Autodesk Fusion 360 part; units mm, degrees
sketch "Sketch1" plane through (0, 0, 0) normal (0, 1, 0) x (1, 0, 0)
  circle A0 centre (0, 0) radius 17 construction
  line L0 (-50, -17) -> (32, -17) construction
  line L1 (32, -17) -> (32, 83) construction
  line L2 (32, 83) -> (-50, 83) construction
  line L3 (-50, 83) -> (-50, -17) construction
  line L4 (-52.028, -78) -> (57.972, -78)
  line L5 (57.972, -78) -> (57.972, -8)
  line L6 (57.972, -8) -> (-52.028, -8)
  line L7 (57.972, -8) -> (32.972, -8)
  line L8 (32.972, -8) -> (32.972, -33)
  line L9 (32.972, -33) -> (57.972, -33)
  line L10 (57.972, -33) -> (57.972, -8)
  line L11 (-52.028, -78) -> (-52.028, -8)
  line L12 (-52.028, -8) -> (57.972, -8)
  line L13 (57.972, -8) -> (57.972, -33)
  line L14 (32.972, -8) -> (57.972, -8)
  line L15 (57.972, -8) -> (57.972, 42)
  line L16 (57.972, 42) -> (32.972, 42)
  line L17 (32.972, 42) -> (32.972, -8)
  line L18 (57.972, 42) -> (-52.028, 42)
  line L19 (-52.028, 42) -> (-52.028, 17)
  line L20 (-52.028, 17) -> (57.972, 17)
  line L21 (57.972, 17) -> (57.972, 42)
  line L22 (-52.028, 17) -> (-52.028, 2)
  line L23 (-52.028, 2) -> (-27.028, 2)
  line L24 (-27.028, 2) -> (-27.028, 17)
  circle A1 centre (-37.028, -63) radius 2.5
  circle A2 centre (42.972, -63) radius 2.5
  circle A3 centre (2.972, -28) radius 2.5
  line L25 (2.972, -78) -> (2.972, -8) construction
  dimension "d1" = 34
  dimension "d2" = 82
  dimension "d3" = 32
  dimension "d4" = 100
  dimension "d5" = 25
  dimension "d6" = 25
  dimension "d7" = 110
  dimension "d8" = 70
  dimension "d9" = 25
  dimension "d10" = 50
  dimension "d11" = 110
  dimension "d12" = 25
  dimension "d13" = 15
  dimension "d14" = 25
  dimension "d15" = 5
  dimension "d16" = 5
  dimension "d17" = 5
  dimension "d18" = 50
  dimension "d19" = 15
  dimension "d20" = 15
  dimension "d21" = 15
  dimension "d22" = 15
extrude "Extrude1" add sketch "Sketch1" along normal blind 10 contours L4 L5 L6 L8 L9 L11 L12 | L5 L6 L7 L8 L9 L10 L12 L13 L14
extrude "Extrude2" add sketch "Sketch1" against normal blind 25 contours L5 L6 L7 L8 L9 L10 L12 L13 L14
extrude "Extrude3" add sketch "Sketch1" along normal blind 25 from surface at -50 contours L5 L6 L7 L8 L9 L10 L12 L13 L14 | L6 L7 L12 L14 L15 L17 L20 | L17 L18 L19 L20 | L15 L16 L17 L18 L20 L21 | L20 L22 L23 L24
chamfer "Chamfer1" distance 20 angle 45 1 edges at (45.472, 0, 33)
fillet "Fillet1" radius 5 4 edges at (57.972, 5, 78) (-52.028, 5, 78) (-52.028, 5, 8) (57.972, -7.5, 8)
fillet "Fillet2" radius 50 1 edges at (45.472, -20, 33)
fillet "Fillet3" radius 5 27 edges at (45.472, -50, 33) (32.972, -50, 8) (2.972, -50, -17) (-27.028, -50, -9.5) (-39.528, -50, -2) (-52.028, -50, -22) (2.972, -50, -42) (57.972, -50, -4.5) (57.972, -25, -14.5) (2.972, -25, -42) (-52.028, -25, -22) (-52.028, -37.5, -2) (-52.028, -37.5, -42) (-39.528, -25, -2) (-27.028, -37.5, -2) (-27.028, -37.5, -17) (2.972, -25, -17) (32.972, -25, -4.5) (32.972, -12.5, 8) (32.972, -2.6777, 50.3223) (32.972, -21.5765, 36.806) (32.972, -45.3553, 33) (57.972, -45.3553, 33) (57.972, -21.5765, 36.806) (57.972, -2.6777, 50.3223) (32.972, -37.5, -17) (-27.028, -25, -9.5)
fillet "Fillet3" radius 5 1 edges at (57.972, -37.5, -42)
fillet "Fillet3" radius 5 7 edges at (-7.028, 0, 8) (-50.5635, 0, 9.4645) (-52.028, 0, 43) (-50.5635, 0, 76.5355) (2.972, 0, 78) (56.5075, 0, 76.5355) (57.972, 0, 63)
fillet "Fillet4" radius 5 5 edges at (34.4365, 1.4645, 9.4645) (32.972, 0, 29.4645) (34.4365, 0, 50.9289) (45.472, 0, 53) (56.5075, 1.4645, 52.3934)
fillet "Fillet5" radius 5 3 edges at (34.4365, -26.4645, 9.4645) (45.472, -25, 8) (56.5075, -26.4645, 9.4645)
equation "d3 = ( ( 34 / 2 ) * 1 mm ) + 15 mm"
Geometry: final body of the model. Coordinates: model frame, mm. A direction names the side the tool comes from. Give positions to 0.01 mm unless a question says otherwise; leave off trailing zeros. Write each loop counter-clockwise with the first axis right and the second up, starting at its lowest first coordinate (ties: lowest second). Pieces come first, ordered by that corner, then holes.
1. Draft query along X for faces 4 (the cylindrical face through (45.28, 4.93, 62.04)), 5 (the cylindrical face through (56.546, -37.395, -40.496)), 6 (the cylindrical face through (4, 2, 77)), 7 (the cylindrical face through (3, -48, -18)). Return one class per face: released by +X, released by -X, zero draft, split by the parting line, or undercut.
2. Section query A-A, the plane z = 63. Return loops of the section in (x, y), then the cut area to 3 significant figures.
3. Line query: probe 1 along X at (y, z) = (6.5, 63); probe 2 along Y at (x, z) = (0.5, 21.5); probe 3 along X at (y, z) = (2.5, 63). Output: solid intervals per line, ascending.
4. Pin query (flat end, axial travel): P1, Ø4.5, axis at x = -37.028, z = 63, coming from the -Y side; P2, Ø1, axis at x = -20, y = 0, coming from the -Z side; P3, Ø20, axis at x = -16.5, z = -20, coming from the +Y side; P4, Ø2, axis at y = -27, z = -6, coming from the +X side. Return the tip coordinate at first contact, or that it passes through.
5. Section query B-B, the plane z = -9. Return loops of the section in (x, y).
6. Section query C-C, the plane x = 51.5. Return loops of the section in (y, z), then the cut area to 3 significant figures.
7. Reachability of faces 1 (the cylindrical face through (34.4, -48.5, 8.3)), 2 (the cylindrical face through (34.4, -42.8, 31.5)), 3 (the cylindrical face through (56.546, 1.504, 64.262)) from +Z, -Z, +X, -X, +Y, -Y: full face, straight path, thin tool, end or side. Return the list, or none.
Computed:
1. face 4: undercut
1. face 5: released by +X
1. face 6: zero draft
1. face 7: undercut
2. outline: (-52.03, 5) arc R5 ccw to (-47.03, 0) - (-39.53, 0) - (-39.53, 10) - (-52.03, 10) - close; (-34.53, 0) - (40.47, 0) - (40.47, 10) - (-34.53, 10) - close; (45.47, 0) - (52.97, 0) arc R5 ccw to (57.97, 5) - (57.97, 10) - (45.47, 10) - close
2. area: 989 mm2
3. probe 1: x = -52.03 to -39.53, -34.53 to 40.47, 45.47 to 57.97
3. probe 2: y = 0 to 10
3. probe 3: x = -51.36 to -39.53, -34.53 to 40.47, 45.47 to 57.3
4. P1: passes through
4. P2: stops at z = 10.82
4. P3: stops at y = -25
4. P4: stops at x = 57.55
5. outline: (-52.03, -45) arc R5 ccw to (-47.03, -50) - (-32.03, -50) arc R5 ccw to (-27.03, -45) - (-27.03, -30) arc R5 ccw to (-32.03, -25) - (-47.03, -25) arc R5 ccw to (-52.03, -30) - close; (32.97, -45) arc R5 ccw to (37.97, -50) - (52.97, -50) arc R5 ccw to (57.97, -45) - (57.97, -30) arc R5 ccw to (52.97, -25) - (37.97, -25) arc R5 ccw to (32.97, -30) - close
6. outline: (-50, -37) arc R5 ccw to (-45, -42) - (-30, -42) arc R5 ccw to (-25, -37) - (-25, 3) arc R5 cw to (-20, 8) - (10, 8) - (10, 78) - (5, 78) arc R5 ccw to (0, 73) - (0, 55.07) arc R5 cw to (-1.46, 51.54) - (-5.36, 47.64) arc R50 cw to (-40.71, 33) - (-45, 33) arc R5 ccw to (-50, 28) - close
6. area: 3,440 mm2
7. face 1: +Z, -Y
7. face 2: +Z, -X, -Y
7. face 3: +Z, +X, -Y
